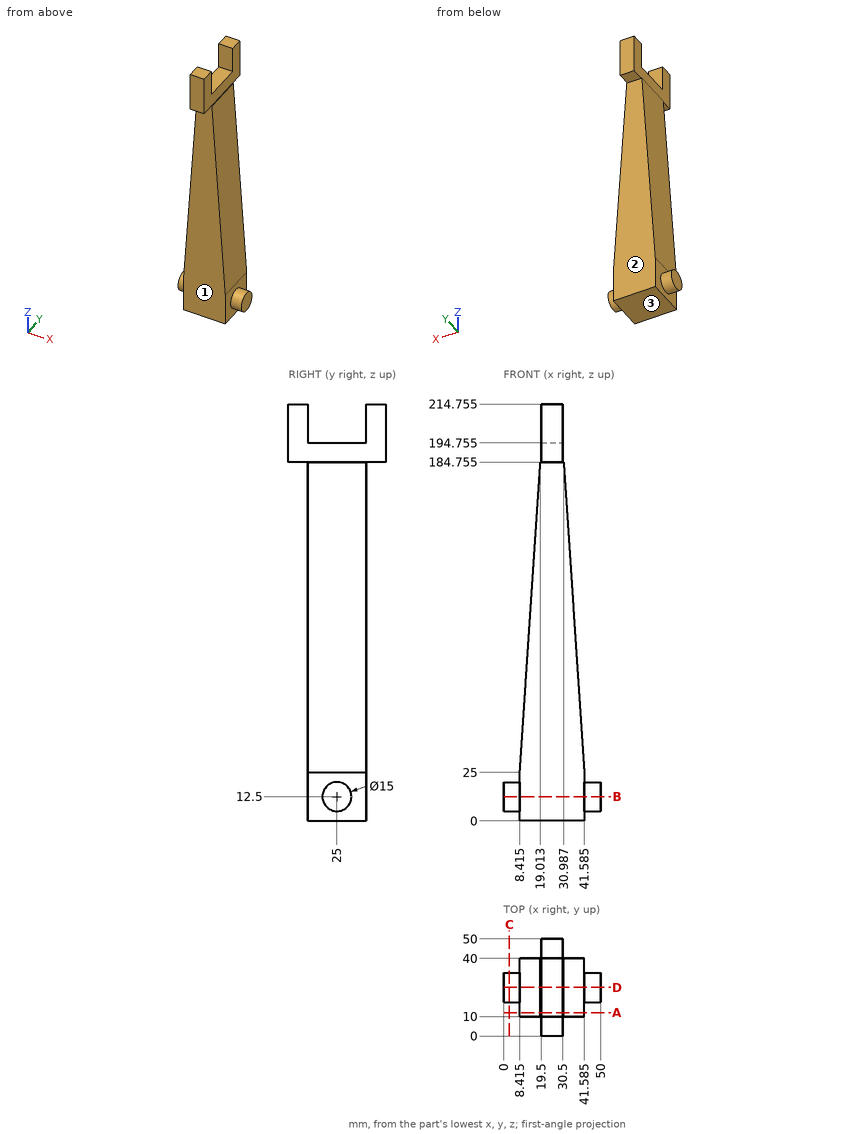
Could you check a few things on this drawing? It's one solid part, dimensions in mm from its lowest x, y, z. A direction names the side the tool comes from. Coordinates: 2 decimals unless noted, no trailing zeros. Loops run counter-clockwise (first coordinate to the right, second up) from the corner with the lowest first, then second, coordinate; pieces in that order, holes last.
1. I need wall thicknesses on L1, parallel to X at y = 11, z = 162; L2, parallel to Y at x = 18, z = 119.5; L3, parallel to X at y = 40.5, z = 199. Which ranges of each line are inside material? Lowest first, please.
2. Imagine slicing it at A-A (y = 12). Please give me the cut outline in (x, z) (1 decimal), and give its area (3 significant figures).
3. For P1, Ø8, axis at y = 14.5, z = 168.5, coming from the -X side; P2, Ø3, axis at x = 24.5, z = 112.5, coming from the +Y side; P3, Ø5.5, axis at x = 24.5, y = 23, coming from the +Z side (3 decimals), each with a flat end and sliding along its axis, tell me the tip position at first contact or that it passes through.
4. Imagine slicing it at C-C (x = 3). Please give me the cut outline in (y, z), and give its area (3 significant figures).
5. Imagine slicing it at D-D (y = 25). Please give me the cut outline in (x, z) (1 decimal), and give its area (3 significant figures).
6. Imagine slicing it at B-B (z = 12.5). Please give me the cut outline in (x, y) (3 decimals).
7. For the marked faces 1, 2 and 3, which set-ups out of +Z, -Z, +X, -X, +Y, -Y let a thin tool reach every point of the face, with its end or its side?
Computed values:
1. L1: x = 17.5 to 32.5
1. L2: y = 10 to 40
1. L3: x = 19.5 to 30.5
2. outline: (8.4, 0) - (41.6, 0) - (41.6, 25) - (31, 184.8) - (30.5, 184.8) - (30.5, 194.8) - (19.5, 194.8) - (19.5, 184.8) - (19, 184.8) - (8.4, 25) - close
2. area: 4,550 mm2
3. P1: stops at x = 17.67
3. P2: stops at y = 40
3. P3: stops at z = 194.755
4. outline: circle Ø15 at (25, 12.5)
4. area: 177 mm2
5. outline: (0, 5) - (8.4, 5) - (8.4, 0) - (41.6, 0) - (41.6, 5) - (50, 5) - (50, 20) - (41.6, 20) - (41.6, 25) - (31, 184.8) - (30.5, 184.8) - (30.5, 194.8) - (19.5, 194.8) - (19.5, 184.8) - (19, 184.8) - (8.4, 25) - (8.4, 20) - (0, 20) - close
5. area: 4,800 mm2
6. outline: (0, 17.5) - (8.415, 17.5) - (8.415, 10) - (41.585, 10) - (41.585, 17.5) - (50, 17.5) - (50, 32.5) - (41.585, 32.5) - (41.585, 40) - (8.415, 40) - (8.415, 32.5) - (0, 32.5) - close
7. face 1: -Z, +X, -X, -Y
7. face 2: -Z, +X, -X, +Y
7. face 3: -Z, +X, -X, +Y, -Y
